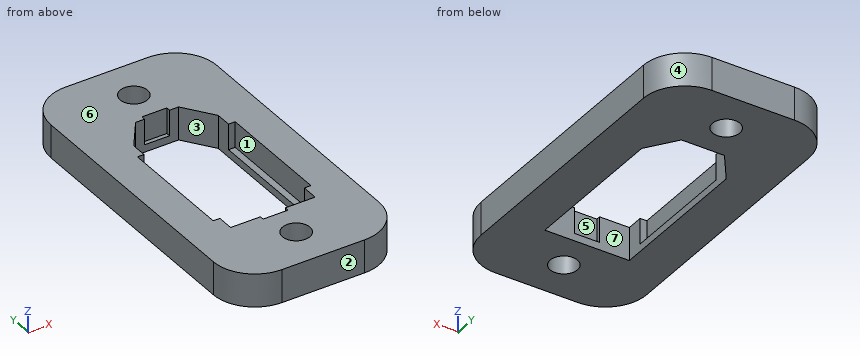
from build123d import *

# Parameters (mm, degrees)
F0_W     = 20
F0_H     = 40
F0_R     = 1.65
F1_DEPTH = 4
F2_R     = 5
F4_W     = 0.8
F4_H     = 14
F4_W_2   = 3
F4_H_2   = 0.5
F5_DEPTH = 3.5


with BuildPart() as f1:
    # F0 (on Top) → F1 (new body)
    with BuildSketch(Plane.XY):
        Rectangle(F0_W, F0_H)
        with Locations((0, -15)):
            Circle(F0_R, mode=Mode.SUBTRACT)
        Polygon((5.1, -10.7), (-5.1, -10.7), (-5.1, 7.2), (-2.6, 10.7), (2.6, 10.7), (5.1, 7.2), align=None, mode=Mode.SUBTRACT)
        with Locations((0, 15)):
            Circle(F0_R, mode=Mode.SUBTRACT)
    extrude(amount=F1_DEPTH)

    # F2
    f2_edges = [f1.edges().sort_by_distance(p)[0] for p in [
        (-10, 20, 2),
        (-10, -20, 2),
        (10, -20, 2),
        (10, 20, 2),
    ]]
    fillet(f2_edges, radius=F2_R)

    # F4 (on offset) → F5 (cut)
    with BuildSketch(Plane.XY.offset(0.9)):
        Polygon((-5.1, -8.7), (-5.1, -10.7), (-1.5, -10.7), (1.5, -10.7), (5.1, -10.7), (5.1, -8.7), (5.1, 5.3), (5.1, 7.2), (2.6, 10.7), (1.5, 10.7), (-1.5, 10.7), (-2.6, 10.7), (-5.1, 7.2), (-5.1, 5.3), align=None)
        with Locations((-5.5, -1.7)):
            Rectangle(F4_W, F4_H)
        with Locations((0, 10.95)):
            Rectangle(F4_W_2, F4_H_2)
        with Locations((5.5, -1.7)):
            Rectangle(F4_W, F4_H)
        with Locations((0, -10.95)):
            Rectangle(F4_W_2, F4_H_2)
    extrude(amount=F5_DEPTH, mode=Mode.SUBTRACT)


solid = f1.part
Model file for the job. Use its own axes, mm. Face numbers are marked on the shaded views. A direction names the side the tool comes from. Round coordinates to 2 decimals unless told otherwise and drop trailing zeros. Loops run counter-clockwise (first coordinate to the right, second up) from the corner with the lowest first, then second, coordinate; pieces in that order, holes last. Notation, with made-up numbers: (7, -0.75) -> (23, -0.75) arc R18 cw to (23, 22.25) -> close; hole circle Ø8 at (-30, 42.25). An arc over 180 degrees is marked (long way). Answer as CSV lines item,"result". Start each with the question number.
1) Tool access for the marked faces 1, 2 and 3: list every direction of +Z, -Z, +X, -X, +Y, -Y with a clear straight run to the whole face (end or side of a thin tool).
2) Pin check, flat tips, straight feed: P1, Ø0.6, axis at x = 5.5, y = -1.5, coming from the +Z side; P2, Ø1, axis at x = 7.5, z = 1, coming from the +Y side; P3, Ø0.6, axis at x = -5.5, z = 1.5, coming from the +Y side. Stop position of each tip, or through.
3) Slice it at A-A (x = 0). List the corners of the cut face in (y, z).
4) Slice it at D-D (y = 16). List the corners of the cut face in (x, z).
5) Probe line 1 along Y through (x, z) = (0, 2.5); line 2 along Y through (x, z) = (1.75, 1); line 3 along X through (y, z) = (-6, 3.2). List the from-to ranges inside material, lowest first.
6) Slice it at B-B (z = 3.45). State how many separate pieces and enclosed holes the cut face has, plus the area to 3 significant figures.
7) Slice it at C-C (x = -3.75). List the corners of the cut face in (y, z).
8) Mould opens along Y. For the marked faces 4, 5, 6 and 7 say: +Y half, -Y half, draft (parallel to the pull), parting line (faces both ways), or undercut.
Filled in:
1,face 1,"+Z"
1,face 2,"+Z, -Z, +X, -X, -Y"
1,face 3,"+Z, -Z"
2,P1,"stops at z = 0.9"
2,P2,"stops at y = 19.58"
2,P3,"stops at y = 20"
3,outline,"(-20, 0) -> (-16.65, 0) -> (-16.65, 4) -> (-20, 4) -> close; (-13.35, 0) -> (-10.7, 0) -> (-10.7, 0.9) -> (-11.2, 0.9) -> (-11.2, 4) -> (-13.35, 4) -> close; (10.7, 0) -> (13.35, 0) -> (13.35, 4) -> (11.2, 4) -> (11.2, 0.9) -> (10.7, 0.9) -> close; (16.65, 0) -> (20, 0) -> (20, 4) -> (16.65, 4) -> close"
4,outline,"(-9.9, 0) -> (-1.31, 0) -> (-1.31, 4) -> (-9.9, 4) -> close; (1.31, 0) -> (9.9, 0) -> (9.9, 4) -> (1.31, 4) -> close"
5,line 1,"y = -20 to -16.65, -13.35 to -11.2, 11.2 to 13.35, 16.65 to 20"
5,line 2,"y = -20 to -10.7, 10.7 to 20"
5,line 3,"x = -10 to -5.9, 5.9 to 10"
6,separate pieces,"1"
6,enclosed holes,"3"
6,area,"527 mm2"
7,outline,"(-20, 0) -> (-10.7, 0) -> (-10.7, 4) -> (-20, 4) -> close; (9.09, 0) -> (20, 0) -> (20, 4) -> (9.09, 4) -> close"
8,face 4,"+Y half"
8,face 5,"undercut"
8,face 6,"draft"
8,face 7,"undercut"
